Autodesk Inventor part; units mm, degrees
ref_plane "YZ Plane" through (0, 0, 0) normal (1, 0, 0) x (0, 1, 0)
ref_plane "XZ Plane" through (0, 0, 0) normal (0, 1, 0) x (-1, 0, 0)
ref_plane "XY Plane" through (0, 0, 0) normal (0, 0, 1) x (1, 0, 0)
sketch "Sketch1" plane through (0, 0, 0) normal (0, 1, 0) x (-1, 0, 0)
  line L0 (86, 229) -> (-74, 229)
  line L1 (-74, 229) -> (-74, -371)
  line L2 (-74, -371) -> (86, -371)
  line L3 (86, -371) -> (86, 229)
  line L4 (86, 229) -> (-74, 229)
  line L5 (-74, 229) -> (-74, 429)
  line L6 (-74, 429) -> (86, 429)
  line L7 (86, 429) -> (86, 229)
  line L8 (-74, 229) -> (86, -371)
  line L9 (-74, 229) -> (63.0532, 429)
  line L10 (-74, 429) -> (-54, 429)
  line L11 (-54, 429) -> (-54, -371)
  line L12 (-54, -371) -> (-74, -371)
  line L13 (-74, -371) -> (-74, 429)
  point P0 (0, 0)
  point P1 (-54, 258.1857)
  point P2 (-54, 154)
  dimension "d0" = 600
  dimension "d1" = 200
  dimension "d2" = 160
  dimension "d3" = 20
extrude "Extrusion1" add sketch "Sketch1" along normal blind 30 contours L3 L8 L11 L0 | L0 L11 L9 L6 L7
sketch "Sketch2" plane through (0, 30, 0) normal (0, 1, 0) x (1, 0, 0)
  line L0 (75.5798, -163.6757) -> (-122, -163.6757)
  line L1 (-122, -163.6757) -> (-122, -153.6757)
  line L2 (-122, -153.6757) -> (75.5798, -153.6757)
  line L3 (75.5798, -153.6757) -> (75.5798, -163.6757)
  line L4 (143.751, -33.6757) -> (-97.1737, -33.6757)
  line L5 (-97.1737, -33.6757) -> (-97.1737, -18.6757)
  line L6 (-97.1737, -18.6757) -> (143.751, -18.6757)
  line L7 (143.751, -18.6757) -> (143.751, -33.6757)
  line L8 (152.9485, -258.6757) -> (-87.9762, -258.6757)
  line L9 (-87.9762, -258.6757) -> (-87.9762, -243.6757)
  line L10 (-87.9762, -243.6757) -> (152.9485, -243.6757)
  line L11 (152.9485, -243.6757) -> (152.9485, -258.6757)
  line L12 (-86, -429) -> (-63.0532, -429)
  line L13 (-63.0532, -429) -> (54, -258.1857)
  line L14 (54, -258.1857) -> (54, -154)
  line L15 (54, -154) -> (-86, 371)
  line L16 (-86, 371) -> (-86, -429)
  line L17 (-76, -419) -> (-68.3232, -419)
  line L18 (-68.3232, -419) -> (44, -255.0882)
  line L19 (44, -255.0882) -> (44, -155.3104)
  line L20 (44, -155.3104) -> (-76, 294.6896)
  line L21 (-76, 294.6896) -> (-76, -419)
  line L22 (38.103, -337.8179) -> (-236.6655, -337.8179)
  line L23 (-236.6655, -337.8179) -> (-236.6655, -322.8179)
  line L24 (-236.6655, -322.8179) -> (38.103, -322.8179)
  line L25 (38.103, -322.8179) -> (38.103, -337.8179)
  line L26 (-19.6002, -33.6757) -> (-9.6002, -33.6757)
  line L27 (-9.6002, -33.6757) -> (-9.6002, -433)
  line L28 (-9.6002, -433) -> (-19.6002, -433)
  line L29 (-19.6002, -433) -> (-19.6002, -33.6757)
  line L30 (-76, -419) -> (-66, -419)
  line L31 (-66, -419) -> (-66, 295.0501)
  line L32 (-66, 295.0501) -> (-76, 295.0501)
  line L33 (-76, 295.0501) -> (-76, -419)
  point P0 (0, 0)
  point P1 (-76, -18.6757)
  point P2 (7.5641, -18.6757)
  point P3 (-76, -33.6757)
  point P4 (-76, -153.6757)
  point P5 (44, -159.6038)
  point P6 (11.5641, -33.6757)
  point P7 (-76, -163.6757)
  point P8 (-76, -243.6757)
  point P9 (38.3772, -263.2935)
  point P10 (44, -163.6757)
  point P11 (41.5416, -258.6757)
  point P12 (-76, -258.6757)
  point P13 (-94.6892, -355.1147)
  point P14 (-104.6892, -352.0171)
  point P15 (43.5641, -153.6757)
  point P16 (44, -243.6757)
  point P17 (-86, -163.6757)
  point P18 (-86, -243.6757)
  point P19 (-86, -33.6757)
  point P20 (-86, -153.6757)
  point P21 (53.9135, -153.6757)
  point P22 (21.9135, -33.6757)
  point P23 (17.9135, -18.6757)
  point P24 (-86, -18.6757)
  point P25 (-86, -258.6757)
  point P26 (54, -163.6757)
  point P27 (-86, -337.8179)
  point P28 (-86, -322.8179)
  point P29 (54, -243.6757)
  point P30 (53.6642, -258.6757)
  point P31 (9.7098, -322.8179)
  point P32 (-0.5692, -337.8179)
  point P33 (-9.6002, -350.9967)
  point P34 (-19.6002, -365.5895)
  point P35 (-66, 257.1896)
  point P36 (-66, -18.6757)
  point P37 (-9.6002, -33.6757)
  point P38 (-9.6002, -153.6757)
  point P39 (-66, -33.6757)
  point P40 (-66, -153.6757)
  point P41 (-19.6002, -153.6757)
  point P42 (-66, -163.6757)
  point P43 (-66, -243.6757)
  point P44 (-19.6002, -243.6757)
  point P45 (-19.6002, -163.6757)
  point P46 (-9.6002, -163.6757)
  point P47 (-9.6002, -243.6757)
  point P48 (-9.6002, -258.6757)
  point P49 (-9.6002, -322.8179)
  point P50 (-2.4129, -322.8179)
  point P51 (-66, -258.6757)
  point P52 (-66, -322.8179)
  point P53 (-19.6002, -322.8179)
  point P54 (-19.6002, -258.6757)
  point P55 (-66, -337.8179)
  point P56 (-66, -415.6098)
  point P57 (-19.6002, -347.8991)
  point P58 (-19.6002, -337.8179)
  dimension "d6" = 10
  dimension "d7" = 15
  dimension "d8" = 15
  dimension "d9" = 120
  dimension "d10" = 80
  dimension "d11" = 10
  dimension "d15" = 15
  dimension "d16" = 10
  dimension "d17" = 20
extrude "Extrusion2" cut sketch "Sketch2" against normal blind 15 contours L19 L10 L27 L0 | L2 L27 L4 L20 | L29 L10 L31 L0 | L2 L31 L4 L29 | L8 L18 L24 L27 | L6 L31 L20 | L29 L24 L31 L8 | L29 L18 L31 L22
properties part number "Nozki" material "Aluminum 6061"
Input: part model. Units: mm. Frame: model coordinates. A direction names the side the tool comes from. Coordinates: 2 decimals unless noted, no trailing zeros. Order: outer loops, then holes, each group sorted by start corner. A loop starts at its lowest first (then second) coordinate and runs counter-clockwise, first axis right, second up.
1. Ray query, line 1 along Y through (x, z) = (-35, 40.5); line 2 along X through (y, z) = (16.5, -29); line 3 along X through (y, z) = (29, 22). Return the intervals inside material, ascending.
Checked values:
line 1: y = 0 to 15
line 2: x = -86 to -66, -5.15 to 5.2
line 3: x = -86 to 18.8
2. Contact query for flat-ended pins moving along their axis: P1, Ø4.5, axis at y = 21.5, z = -90.5, coming from the +X side; P2, Ø4.5, axis at y = 23.5, z = 363.5, coming from the +X side; P3, Ø8, axis at x = -61, z = 151.5, coming from the +Y side; P4, Ø4.5, axis at y = 25.5, z = 86.5, coming from the +X side. Output: stop coordinate, or through.
Checked values:
P1: stops at x = -10.6
P2: stops at x = -16.63
P3: stops at y = 30
P4: stops at x = 36.6
3. Cut plane A-A, the plane z = 211.5. Return loops of the section in (x, y), plus the area to 3 significant figures.
Checked values:
outline: (-86, 0) - (54, 0) - (54, 30) - (44, 30) - (44, 15) - (-9.6, 15) - (-9.6, 30) - (-19.6, 30) - (-19.6, 15) - (-66, 15) - (-66, 30) - (-86, 30) - close
area: 2,700 mm2
4. Cut plane B-B, the plane x = -38.5. Return loops of the section in (y, z) (3 decimals).
Checked values:
outline: (0, -192.875) - (30, -192.875) - (30, -154.065) - (15, -154.065) - (15, 18.676) - (30, 18.676) - (30, 33.676) - (15, 33.676) - (15, 153.676) - (30, 153.676) - (30, 163.676) - (15, 163.676) - (15, 243.676) - (30, 243.676) - (30, 258.676) - (15, 258.676) - (15, 322.818) - (30, 322.818) - (30, 337.818) - (15, 337.818) - (15, 375.479) - (30, 375.479) - (30, 393.17) - (0, 393.17) - close
5. Access query for faces 5 (the flat face through (-31, 0, 123)), 6 (the flat face through (-43, 15, 93)). Directions: +Z, -Z, +X, -X, +Y, -Y. A direction counts if a zero-diameter tool reaches every point of the face in a straight line with its end or side. Return the directions, or none.
Checked values:
face 5: +Z, -Z, +X, -X, -Y
face 6: +Y
6. Cut plane D-D, the plane z = -183. Return loops of the section in (x, y), plus the area to 3 significant figures.
Checked values:
outline: (-86, 0) - (-35.87, 0) - (-35.87, 30) - (-46.22, 30) - (-46.22, 15) - (-66, 15) - (-66, 30) - (-86, 30) - close
area: 1,210 mm2
7. Cut plane C-C, the plane y = 9.75. Return loops of the section in (x, z).
Checked values:
outline: (-86, -371) - (54, 154) - (54, 258.19) - (-63.05, 429) - (-86, 429) - close
8. Draft query along X for faces 1 (the flat face through (-3.71, 14.79, 342.4)), 2 (the flat face through (18, 23, 163.676)), 3 (the flat face through (-68, 30, 90)), 4 (the flat face through (-42, 23, 33.676)). Return one class per face: +X half, -X half, draft (parallel to the pull), parting line (faces both ways), or undercut.
Checked values:
face 1: +X half
face 2: undercut
face 3: draft
face 4: undercut
